Design review of the part built by this model. Coordinates are the model's own, in mm. A direction names the side the tool comes from. Round coordinates to 2 decimals unless told otherwise and drop trailing zeros. Order: outer loops, then holes, each group sorted by start corner. A loop starts at its lowest first (then second) coordinate and runs counter-clockwise, first axis right, second up. Notation, with made-up numbers: M -25.5,25.25 L -14.5,25.25 A22 cw -14.5,57.25 Z; hole C 13,52 d7. An arc over 180 degrees is marked long. Use a Markdown table: item, result. Add a question column.
(1) Take a section at A-A (x = 0). Write out the cut boundary in (y, z).
(2) To check wall thickness, follow probe 1 along X at (y, z) = (21.25, 0); probe 2 along Z at (x, y) = (8.5, 5.5); probe 3 along Y at (x, z) = (0, 6.4). State the ranges of each line that lie inside material, in increasing order. Write a range as from..to.
(3) For pin 1 (1.2 mm diameter, centred on x = -1.5, z = -9.5, fed in from -Y); pin 2 (4.5 mm diameter, centred on x = 1.5, y = 8, fed in from -Z); pin 3 (1.4 mm diameter, centred on x = -9, y = 11, fed in from -Z), all flat-tipped, find the tip position at first contact; note any pin that passes through.
(4) Take a section at D-D (y = 13). Write out the cut boundary in (x, z), then the cut area to 3 significant figures.
(5) Take a section at B-B (z = 0). Write out the cut boundary in (x, y).
(6) Machinability: for faces 4 (the face through (0, 18, 9)), 5 (the face through (-4, 9, -5.25)), 6 (the face through (0, 0, -7)), 7 (the face through (0, 18, -9)), 8 (the face through (-6.097, 14.217, 6.027)), which of the approach directions +Z, -Z, +X, -X, +Y, -Y give a long, thin tool a straight path to every point of the face, cutting with its end or side? Answer none if there is none.
(7) Take a section at C-C (y = 7.5). Write out the cut boundary in (x, z).
(8) The part is to be moulded in two halves that separate along X. For faces 1 (the face through (-3, 7.6, 6.9)), 2 (the face through (-9, 9, 5.25)), 3 (the face through (10.906, 19.006, -1.432)), say which applies: released by +X, released by -X, zero draft, split by the parting line, or undercut.
```python
from build123d import *

# Parameters (mm, degrees)
SKETCH_2_R          = 11
EXTRUDE_1_DEPTH     = 23
CUT_EXTRUDE_START   = -8.5
SKETCH_3_W          = 30
SKETCH_3_H          = 18
CUT_EXTRUDE_1_DEPTH = 20.266886754
CUT_EXTRUDE_START_2 = 8.5
SKETCH_3_5_W        = 30
SKETCH_3_5_H        = 18
CUT_EXTRUDE_2_DEPTH = 20.266886754
SKETCH_3_6_W        = 30
SKETCH_3_6_H        = 18
CUT_EXTRUDE_3_DEPTH = 5.25
SKETCH_4_R          = 3
CUT_EXTRUDE_4_DEPTH = 33.097507691
SKETCH_6_R          = 1.5
CUT_EXTRUDE_5_DEPTH = 28.766886754
SKETCH_8_R          = 1.5
CUT_EXTRUDE_6_DEPTH = 28.766886754


with BuildPart() as part:
    # Sketch 2 → Extrude 1 (new body)
    with BuildSketch(Plane(origin=(0, 0, 0), x_dir=(1, 0, 0), z_dir=(0, 1, 0))):
        with Locations(Location((0, 0, 0), (0, 0, 270))):
            Circle(SKETCH_2_R)
    extrude(amount=EXTRUDE_1_DEPTH)

    # Sketch 3 → Cut-Extrude 1 (cut, through all)
    with BuildSketch(Plane.XY.offset(CUT_EXTRUDE_START)):
        with Locations((4, 9)):
            Rectangle(SKETCH_3_W, SKETCH_3_H)
    extrude(amount=-CUT_EXTRUDE_1_DEPTH, mode=Mode.SUBTRACT)

    # Sketch 3_5 → Cut-Extrude 2 (cut, through all)
    with BuildSketch(Plane.XY.offset(CUT_EXTRUDE_START_2)):
        with Locations((4, 9)):
            Rectangle(SKETCH_3_5_W, SKETCH_3_5_H)
    extrude(amount=CUT_EXTRUDE_2_DEPTH, mode=Mode.SUBTRACT)

    # Sketch 3_6 → Cut-Extrude 3 (cut, symmetric)
    with BuildSketch(Plane.XY):
        with Locations((4, 9)):
            Rectangle(SKETCH_3_6_W, SKETCH_3_6_H)
    extrude(amount=CUT_EXTRUDE_3_DEPTH, both=True, mode=Mode.SUBTRACT)

    # Sketch 4 → Cut-Extrude 4 (cut, through all)
    with BuildSketch(Plane.XY.offset(8.5)):
        with Locations((0, 7.5)):
            Circle(SKETCH_4_R)
    extrude(amount=-CUT_EXTRUDE_4_DEPTH, mode=Mode.SUBTRACT)

    # Sketch 6 → Cut-Extrude 5 (cut, through all)
    with BuildSketch(Plane(origin=(0, 23, 0), x_dir=(1, 0, 0), z_dir=(0, 1, 0))):
        with Locations(Location((0, 0, 0), (0, 0, 270))):
            Circle(SKETCH_6_R)
    extrude(amount=-CUT_EXTRUDE_5_DEPTH, mode=Mode.SUBTRACT)

    # Sketch 8 → Cut-Extrude 6 (cut, through all)
    with BuildSketch(Plane(origin=(0, 23, 0), x_dir=(1, 0, 0), z_dir=(0, 1, 0))):
        with Locations(Location((-6.547985936, -4.596072256, 0), (0, 0, 270))):
            Circle(SKETCH_8_R)
        with Locations(Location((6.547985936, 4.596072256, 0), (0, 0, 270))):
            Circle(SKETCH_8_R)
    extrude(amount=-CUT_EXTRUDE_6_DEPTH, mode=Mode.SUBTRACT)


solid = part.part
```
Verdict:
| question | item | result |
|---|---|---|
| 1 | outline | M 0,-8.5 L 4.5,-8.5 L 4.5,-5.25 L 0,-5.25 Z; M 0,5.25 L 4.5,5.25 L 4.5,8.5 L 0,8.5 Z; M 10.5,-8.5 L 18,-8.5 L 18,-11 L 23,-11 L 23,-1.5 L 18,-1.5 L 18,-5.25 L 10.5,-5.25 Z; M 10.5,5.25 L 18,5.25 L 18,1.5 L 23,1.5 L 23,11 L 18,11 L 18,8.5 L 10.5,8.5 Z |
| 2 | probe 1 | x = -11..-1.5, 1.5..11 |
| 2 | probe 2 | z = -6.98..-5.25, 5.25..6.98 |
| 2 | probe 3 | y = 0..4.5, 10.5..23 |
| 3 | pin 1 | stops at y = 18 |
| 3 | pin 2 | stops at z = -8.5 |
| 3 | pin 3 | stops at z = -7.22 |
| 4 | outline | M -9.67,-5.25 A11 ccw -6.98,-8.5 L 6.98,-8.5 A11 ccw 9.67,-5.25 L 7.9,-5.25 A1.5 cw 5.2,-5.25 Z; M -9.67,5.25 L -7.9,5.25 A1.5 cw -5.2,5.25 L 9.67,5.25 A11 ccw 6.98,8.5 L -6.98,8.5 A11 ccw Z |
| 4 | area | 107 mm^2 |
| 5 | outline | M -11,18 L -1.5,18 L -1.5,23 L -11,23 Z; M 1.5,18 L 11,18 L 11,23 L 1.5,23 Z |
| 6 | face 4 | +Z, +X, -X, -Y |
| 6 | face 5 | +X, -X, -Y |
| 6 | face 6 | +Z, -Z, +X, -X, -Y |
| 6 | face 7 | -Z, +X, -X, -Y |
| 6 | face 8 | +Y, -Y |
| 7 | outline | M -9.67,-5.25 A11 ccw -6.98,-8.5 L -3,-8.5 L -3,-5.25 Z; M -9.67,5.25 L -7.9,5.25 A1.5 cw -5.2,5.25 L -3,5.25 L -3,8.5 L -6.98,8.5 A11 ccw Z; M 3,-8.5 L 6.98,-8.5 A11 ccw 9.67,-5.25 L 7.9,-5.25 A1.5 cw 5.2,-5.25 L 3,-5.25 Z; M 3,5.25 L 9.67,5.25 A11 ccw 6.98,8.5 L 3,8.5 Z |
| 8 | face 1 | undercut |
| 8 | face 2 | zero draft |
| 8 | face 3 | split by the parting line |
